Autodesk Inventor part; units mm, degrees
ref_plane "Work Plane1" through (0, 0, 0) normal (1, 0, 0) x (0, 1, 0)
ref_plane "Work Plane2" through (0, 0, 0) normal (0, 0, 1) x (1, 0, 0)
ref_plane "XZ Plane" through (0, 0, 0) normal (0, 1, 0) x (-1, 0, 0)
ref_plane "Work Plane1" through (0, 0, 0) normal (1, 0, 0) x (0, 1, 0)
ref_plane "Work Plane2" through (0, 0, 0) normal (0, 0, 1) x (1, 0, 0)
sketch "Sketch1" plane through (0, 0, 0) normal (0, 1, 0) x (-1, 0, 0)
  circle A0 centre (0, 0) radius 80
  circle A1 centre (0, 0) radius 77.5
  dimension "d0" = 160
  dimension "d1" = 155
extrude "Extrusion1" add sketch "Sketch1" along normal blind 200
sketch "Sketch2" plane through (0, 0, 0) normal (0, 1, 0) x (-1, 0, 0)
  circle A0 centre (0, 0) radius 77.5
  dimension "d4" = 155
extrude "Extrusion2" add sketch "Sketch2" along normal blind 10
sketch "Sketch3" plane through (0, 10, 0) normal (0, 1, 0) x (1, 0, 0)
  circle A0 centre (0, 0) radius 80
  line L0 (79.6477, -7.5) -> (-79.6477, -7.5)
  line L1 (-79.6477, -7.5) -> (-79.6477, 7.5)
  line L2 (-79.6477, 7.5) -> (79.6477, 7.5)
  line L3 (79.6477, 7.5) -> (79.6477, -7.5)
  line L4 (79.6477, -7.5) -> (-79.6477, 7.5) construction
  line L5 (-79.6477, -7.5) -> (79.6477, 7.5) construction
  line L6 (7.5, -76) -> (-7.5, -76)
  line L7 (-7.5, -76) -> (-7.5, 76)
  line L8 (-7.5, 76) -> (7.5, 76)
  line L9 (7.5, 76) -> (7.5, -76)
  line L10 (7.5, -76) -> (-7.5, 76) construction
  line L11 (-7.5, -76) -> (7.5, 76) construction
  point P0 (-7.5, 7.5)
  point P1 (-7.5, -7.5)
  point P2 (7.5, -7.5)
  point P3 (7.5, 7.5)
  dimension "d7" = 15
  dimension "d8" = 15
  dimension "d9" = 152
extrude "Extrusion3" add sketch "Sketch3" along normal blind 190 contours L3 L0 L9 L2 | L2 L7 L0 L1 | L9 L0 L7 L2 | L2 L7 L8 L9 | L9 L6 L7 L0
sketch "Sketch4" plane through (0, 0, 0) normal (0, -1, 0) x (1, 0, 0)
  circle A0 centre (0, 0) radius 2.5
  dimension "d14" = 5
extrude "Extrusion4" cut sketch "Sketch4" against normal blind 190
sketch "Sketch5" plane through (0, 200, 0) normal (0, 1, 0) x (1, 0, 0)
  line L0 (7.5, 76) -> (7.5, 7.5)
  line L1 (-7.5, -76) -> (7.5, -76)
  line L2 (7.5, -76) -> (7.5, 76)
  line L3 (7.5, 76) -> (-7.5, 76)
  line L4 (-7.5, 76) -> (-7.5, -76)
  circle A0 centre (0, 0) radius 2.5
  line L5 (-7.5, -76) -> (7.5, 76) construction
  line L6 (7.5, -76) -> (-7.5, 76) construction
  line L7 (-77.1362, 7.5) -> (77.1362, 7.5)
  line L8 (77.1362, 7.5) -> (77.1362, -7.5)
  line L9 (77.1362, -7.5) -> (-77.1362, -7.5)
  line L10 (-77.1362, -7.5) -> (-77.1362, 7.5)
  line L11 (-77.1362, 7.5) -> (77.1362, -7.5) construction
  line L12 (77.1362, 7.5) -> (-77.1362, -7.5) construction
  point P0 (-7.5, 7.5)
  point P1 (-7.5, -7.5)
  point P2 (7.5, -7.5)
extrude "Extrusion5" cut sketch "Sketch5" against normal blind 10 contours L0 L7 L4 L3 | L7 L8 L9 L2 | L2 L9 L4 L7 | L2 L1 L4 L9 | L4 L9 L10 L7 | A0
properties part number "aa"
Input: part model. Units: mm. Frame: model coordinates. A direction names the side the tool comes from. Coordinates: 2 decimals unless noted, no trailing zeros. Order: outer loops, then holes, each group sorted by start corner. A loop starts at its lowest first (then second) coordinate and runs counter-clockwise, first axis right, second up. Notation, with made-up numbers: M -33.75,7.5 L -20.75,7.5 A24 cw -20.75,37.5 Z; hole C 70.5,86.5 d1. An arc over 180 degrees is marked long. Answer in a Markdown table with one row per item.
(1) Draft query along X for faces 3 (the flat face through (-17, 0, 1)), 4 (the flat face through (-16, 10, 35)), 5 (the cylindrical face through (17.34, 98.6, 78.1)). Return one class per face: pulls with the +X half, pulls with the -X half, needs draft (parallel to the pull), parting line crosses it, or undercut.
Numbers:
| item | result |
|---|---|
| face 3 | needs draft |
| face 4 | undercut |
| face 5 | parting line crosses it |
(2) Access query for faces 1 (the flat face through (-77.136, 195, 0)), 2 (the flat face through (66, 200, 42)). Directions: +Z, -Z, +X, -X, +Y, -Y. A direction counts if a zero-diameter tool reaches every point of the face in a straight line with its end or side. Return the directions, or none.
Numbers:
| item | result |
|---|---|
| face 1 | +Y |
| face 2 | +Z, -Z, +X, -X, +Y |
(3) Contact query for flat-ended pins moving along their axis: pin 1 Ø21 at (x, y) = (-53, 125) entering from -Z; pin 2 Ø6 at (x, y) = (-34.5, 113) entering from +Z; pin 3 Ø8 at (x, y) = (-49.5, 120) entering from -Z. Output: stop coordinate, or through.
Numbers:
| item | result |
|---|---|
| pin 1 | stops at z = -67.78 |
| pin 2 | stops at z = 73.54 |
| pin 3 | stops at z = -65.8 |
(4) Section query A-A, the plane x = 0. Output: boundary loops of the cut face in (y, z), plus the area to 3 significant figures.
Numbers:
| item | result |
|---|---|
| outline | M 0,-80 L 200,-80 L 200,-77.5 L 10,-77.5 L 10,-76 L 190,-76 L 190,-2.5 L 0,-2.5 Z; M 0,2.5 L 190,2.5 L 190,76 L 10,76 L 10,77.5 L 200,77.5 L 200,80 L 0,80 Z |
| area | 29,000 mm^2 |
(5) Section query D-D, the plane x = 55. Output: boundary loops of the cut face in (y, z).
Numbers:
| item | result |
|---|---|
| outline | M 0,-58.09 L 200,-58.09 L 200,-54.6 L 10,-54.6 L 10,-7.5 L 190,-7.5 L 190,7.5 L 10,7.5 L 10,54.6 L 200,54.6 L 200,58.09 L 0,58.09 Z |
(6) Section query C-C, the plane z = 0. Output: boundary loops of the cut face in (x, y).
Numbers:
| item | result |
|---|---|
| outline | M -80,0 L -2.5,0 L -2.5,190 L -77.14,190 L -77.14,200 L -80,200 Z; M 2.5,0 L 80,0 L 80,200 L 77.14,200 L 77.14,190 L 2.5,190 Z |
(7) Section query B-B, the plane y = 174.5. Output: boundary loops of the cut face in (x, z).
Numbers:
| item | result |
|---|---|
| outline | C 0,0 d160; hole M -77.14,-7.5 A77.5 ccw 77.14,-7.5 L 7.5,-7.5 L 7.5,-76 L -7.5,-76 L -7.5,-7.5 Z; hole M -77.14,7.5 L -7.5,7.5 L -7.5,76 L 7.5,76 L 7.5,7.5 L 77.14,7.5 A77.5 ccw Z; hole C 0,0 d5 |
(8) Material intervals for line 1 (Z direction, x = 0, y = 44); line 2 (Z direction, x = 35, y = 102); line 3 (X direction, y = 50, z = 39), sorted ascending. Write a range as [from, to].
Numbers:
| item | result |
|---|---|
| line 1 | z = [-80, -77.5], [-76, -2.5], [2.5, 76], [77.5, 80] |
| line 2 | z = [-71.94, -69.15], [-7.5, 7.5], [69.15, 71.94] |
| line 3 | x = [-69.85, -66.97], [-7.5, 7.5], [66.97, 69.85] |
